The model under review builds one solid part; all positions refer to its coordinate system, in mm. Face numbers are marked on the shaded views. Round coordinates to 2 decimals unless told otherwise and drop trailing zeros. Write each loop counter-clockwise with the first axis right and the second up, starting at its lowest first coordinate (ties: lowest second). Pieces come first, ordered by that corner, then holes.
Item 1: To check wall thickness, follow L1, parallel to X at y = 23.5, z = 1.65; L2, parallel to X at y = 20.5, z = 1.75; L3, parallel to X at y = -9.5, z = 1. State the ranges of each line that lie inside material, in increasing order.
Item 2: Clearance check with flat-ended pins moving along their axes: pin 1 Ø10 at (x, y) = (37.5, -20) entering from +Z; pin 2 Ø3 at (x, z) = (-10, -1) entering from +Y; pin 3 Ø1.4 at (x, z) = (-72.5, 1) entering from +Y; pin 4 Ø4 at (y, z) = (-5, 3) entering from +X. State where each tip first meets the part, or that it passes through.
Item 3: Add section B-B (z = 1.65). Give the boundary of the cut face in (x, y).
Item 4: Add section D-D (y = -12). Give the boundary of the cut face in (x, z).
Item 5: Add section C-C (x = 0). Give the boundary of the cut face in (y, z).
Item 6: Draft analysis for pull direction X (two halves, no side actions). For the marked faces 1 and 2, state which applies: +X half, -X half, draft (parallel to the pull), parting line (faces both ways), or undercut.
Item 7: Add section A-A (y = -36). Give the boundary of the cut face in (x, z).
```python
from build123d import *

# Parameters (mm, degrees)
BOSS_EXTRUDE1_DEPTH = 3.3
CUT_EXTRUDE1_DEPTH  = 3.3
SCALE1_SCALE        = 1.9329
SCALE2_SCALE        = 1.5


with BuildPart() as part:
    # Sketch1 → Boss-Extrude1 (new body)
    with BuildSketch(Plane.XY):
        with BuildLine():
            Line((-26, 0), (-24, 0))
            ThreePointArc((-24, 0), (0, -24), (24, 0))
            Line((24, 0), (26, 0))
            ThreePointArc((26, 0), (0, -26), (-26, 0))
        make_face()
    extrude(amount=BOSS_EXTRUDE1_DEPTH)

    # Sketch2 → Cut-Extrude1 (cut)
    with BuildSketch(Plane(origin=(0, 0, 0), x_dir=(1, 0, 0), z_dir=(0, 1, 0))):
        with BuildLine():
            ThreePointArc((24.5, -1.65), (25, -2.15), (25.5, -1.65))
            Line((25.5, -1.65), (24.5, -1.65))
        make_face()
        with BuildLine():
            Line((24.5, -1.65), (25.5, -1.65))
            ThreePointArc((25.5, -1.65), (25, -1.15), (24.5, -1.65))
        make_face()
        with BuildLine():
            ThreePointArc((-25.5, -1.65), (-25, -2.15), (-24.5, -1.65))
            Line((-24.5, -1.65), (-25.5, -1.65))
        make_face()
        with BuildLine():
            Line((-25.5, -1.65), (-24.5, -1.65))
            ThreePointArc((-24.5, -1.65), (-25, -1.15), (-25.5, -1.65))
        make_face()
    extrude(amount=-CUT_EXTRUDE1_DEPTH, mode=Mode.SUBTRACT)


with BuildPart() as part_1:
    # Scale1: scaled about (0, -16.068164215, 1.65)
    add(part.part.scale(SCALE1_SCALE).moved(Location((0, 14.989990396, -1.539285))))


with BuildPart() as part_2:
    # Scale2: scaled about (0, -16.068164215, 1.65)
    add(part_1.part.scale(SCALE2_SCALE).moved(Location((0, 8.034082107, -0.825))))


solid = part_2.part
```
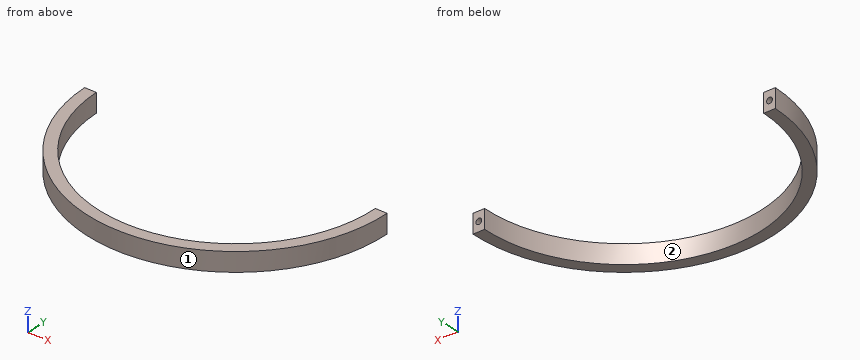
Numbers:
1. L1: x = -75.06 to -73.93, -71.03 to -69.23, 69.23 to 71.03, 73.93 to 75.06
1. L2: x = -74.71 to -68.86, 68.86 to 74.71
1. L3: x = -63.88 to -56.93, 56.93 to 63.88
2. pin 1: passes through
2. pin 2: stops at y = -38.11
2. pin 3: stops at y = 20.95
2. pin 4: stops at x = 67.52
3. outline: (-75.38, 30.52) arc R75.38 ccw to (75.38, 30.52) - (73.93, 30.52) - (73.93, 20.95) - (71.03, 20.95) - (71.03, 30.52) - (69.58, 30.52) arc R69.58 cw to (-69.58, 30.52) - (-71.03, 30.52) - (-71.03, 20.95) - (-73.93, 20.95) - (-73.93, 30.52) - close
4. outline: (-62.25, -3.13) - (-55.08, -3.13) - (-55.08, 6.43) - (-62.25, 6.43) - close; (55.08, -3.13) - (62.25, -3.13) - (62.25, 6.43) - (55.08, 6.43) - close
5. outline: (-44.86, -3.13) - (-39.07, -3.13) - (-39.07, 6.43) - (-44.86, 6.43) - close
6. face 1: parting line
6. face 2: undercut
7. outline: (-35.47, -3.13) - (-20.43, -3.13) - (-20.43, 6.43) - (-35.47, 6.43) - close; (20.43, -3.13) - (35.47, -3.13) - (35.47, 6.43) - (20.43, 6.43) - close
